Job drawing, mm, ordinate dimensions from the low corner. One solid piece. Give positions to 0.01 mm unless a question says otherwise; leave off trailing zeros. Write each loop counter-clockwise with the first axis right and the second up, starting at its lowest first coordinate (ties: lowest second). Pieces come first, ordered by that corner, then holes. Notation, with made-up numbers: (11, 11) -> (40, 11) arc R18 cw to (40, 46) -> close; hole circle Ø3 at (45.25, -30). An arc over 180 degrees is marked (long way). Put each result on its own line as item: value. Start each with the question number.
Item 1: Slice it at A-A, the plane z = 31. List the corners of the cut face in (x, y), plus the area to 3 significant figures.
Item 2: Drill centre lines: line 1 along Y through (x, z) = (2, 31); line 2 along Y through (x, z) = (1.5, 35); line 3 along Y through (x, z) = (2.25, 58.5). Where is each one in solid material? Low to high.
Item 3: Slice it at C-C, the plane z = 50.5. List the corners of the cut face in (x, y).
Item 4: Slice it at D-D, the plane x = 1.9. Give the number of separate pieces and of enclosed holes in the cut face, plus the area to 3 significant figures.
Item 5: Slice it at B-B, the plane y = 33.5. List the corners of the cut face in (x, z).
Item 6: Flat gauge pins, fed straight in: pin 1 Ø1.5 at (x, y) = (1.5, 54) entering from -Z; pin 2 Ø0.9 at (x, z) = (1, 53.5) entering from -Y; pin 3 Ø0.9 at (x, y) = (1.5, 67) entering from -Z; pin 4 Ø1.5 at (x, z) = (0.5, 9.5) entering from +Y. Where does each tip first touch, or does it go through?
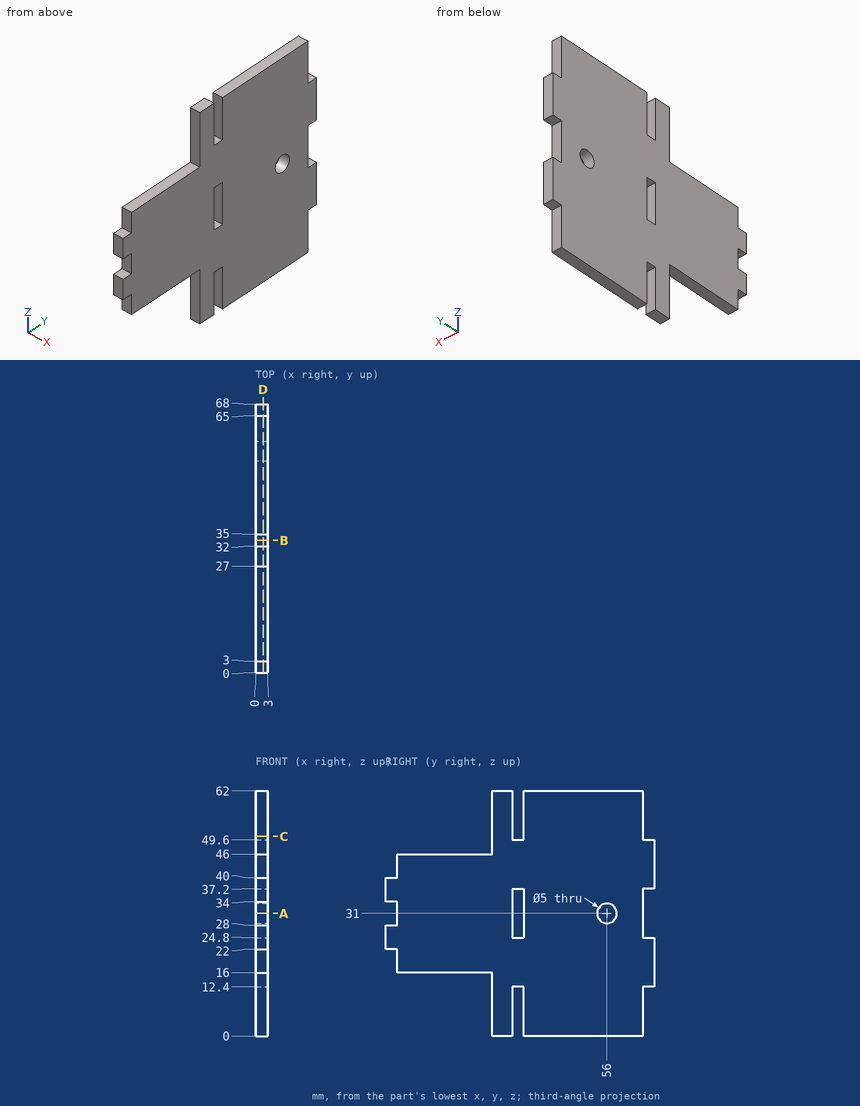
Values follow:
1. outline: (0, 3) -> (3, 3) -> (3, 32) -> (0, 32) -> close; (0, 35) -> (3, 35) -> (3, 53.5) -> (0, 53.5) -> close; (0, 58.5) -> (3, 58.5) -> (3, 65) -> (0, 65) -> close
1. area: 162 mm2
2. line 1: 3 to 32, 35 to 53.5, 58.5 to 65
2. line 2: 0 to 32, 35 to 65
2. line 3: 27 to 32, 35 to 65
3. outline: (0, 27) -> (3, 27) -> (3, 32) -> (0, 32) -> close; (0, 35) -> (3, 35) -> (3, 65) -> (0, 65) -> close
4. separate pieces: 1
4. enclosed holes: 2
4. area: 3,060 mm2
5. outline: (0, 12.4) -> (3, 12.4) -> (3, 24.8) -> (0, 24.8) -> close; (0, 37.2) -> (3, 37.2) -> (3, 49.6) -> (0, 49.6) -> close
6. pin 1: z = 0
6. pin 2: y = 27
6. pin 3: z = 12.4
6. pin 4: y = 65
